from build123d import *

# Parameters (mm, degrees)
BOSS_EXTRUDE1_DEPTH              = 7.62
SKETCH2_W                        = 15.24
SKETCH2_H                        = 10.31875
CUT_EXTRUDE1_DEPTH               = 2.38125
SKETCH4_W                        = 10.31875
SKETCH4_H                        = 15.24
CUT_EXTRUDE2_DEPTH               = 2.38125
CHAMFER1_SIZE                    = 5.08
F_11_32_0_34375_DIAMETER_HOLE1_D = 8.73125


with BuildPart() as part:
    # Sketch1 → Boss-Extrude1 (new body, symmetric)
    with BuildSketch(Plane.XY):
        Polygon((0, 0), (0, 25.4), (6.35, 25.4), (6.35, 6.35), (25.4, 6.35), (25.4, 0), align=None)
    extrude(amount=BOSS_EXTRUDE1_DEPTH, both=True)

    # Sketch2 → Cut-Extrude1 (cut)
    with BuildSketch(Plane(origin=(6.35, 0, 0), x_dir=(0, 0, -1), z_dir=(1, 0, 0))):
        with Locations((0, 20.240625)):
            Rectangle(SKETCH2_W, SKETCH2_H)
    extrude(amount=-CUT_EXTRUDE1_DEPTH, mode=Mode.SUBTRACT)

    # Sketch4 → Cut-Extrude2 (cut)
    with BuildSketch(Plane(origin=(0, 6.35, 0), x_dir=(1, 0, 0), z_dir=(0, 1, 0))):
        with Locations((20.240625, 0)):
            Rectangle(SKETCH4_W, SKETCH4_H)
    extrude(amount=-CUT_EXTRUDE2_DEPTH, mode=Mode.SUBTRACT)

    # Chamfer1
    chamfer1_edges = [part.edges().sort_by_distance(p)[0] for p in [
        (0, 0, 0),
    ]]
    chamfer(chamfer1_edges, length=CHAMFER1_SIZE)

    # 11/32 (0.34375) Diameter Hole1 (through all)
    with Locations(Plane(origin=(2.54, 2.54, 0), x_dir=(0, 0, 1), z_dir=(-0.707106781, -0.707106781, 0))):
        with Locations((0, 0)):
            Hole(F_11_32_0_34375_DIAMETER_HOLE1_D / 2)


solid = part.part
For this review, take the finished solid that the model builds, in its own axes (mm). A direction names the side the tool comes from. Round coordinates to 2 decimals unless told otherwise and drop trailing zeros. Order: outer loops, then holes, each group sorted by start corner. A loop starts at its lowest first (then second) coordinate and runs counter-clockwise, first axis right, second up. Notation, with made-up numbers: (-4, 25) -> (46, 25) arc R16 cw to (46, 38) -> close; hole circle Ø7 at (15.5, 36.5). An arc over 180 degrees is marked (long way). Write item = value, one per line. Start each with the question number.
1) The part is to be moulded in two halves that separate along Y. For faces 3 (the face through (2.58, 2.5, -5.66)), 4 (the face through (2.224, 8.346, 0.568)), 5 (the face through (15.081, 5, 0)), say which applies: +Y half, -Y half, draft (parallel to the pull), parting line (faces both ways), or undercut.
2) Take a section at A-A on z = 5.25. State the section outline as (x, y) points.
3) Tool access review of faces 1 (the face through (20, 3.969, 0)), 2 (the face through (2.58, 2.5, 5.59)): name each direction out of +Z, -Z, +X, -X, +Y, -Y from which nothing blocks a thin tool from reaching the whole face with its end or side.
4) Take a section at C-C on y = 21. State the section outline as (x, z) points, plus the area to 3 significant figures.
5) To check wall thickness, follow line 1 (Y direction, x = 17, z = -3.25); line 2 (X direction, y = 13.5, z = 2.75). State the ranges of each line that lie inside material, in increasing order. Write a range as from..to.
6) Take a section at B-B on z = -0.25. State the section outline as (x, y) points, plus the area to 3 significant figures.
7) Insertion check: pin 1 (2 mm diameter, centred on x = 13.5, y = 7, fed in from +Z); pin 2 (1 mm diameter, centred on y = 5, z = 0.5, fed in from -X); pin 3 (2.5 mm diameter, centred on x = 9.5, z = -1, fed in from +Y); pin 4 (1.5 mm diameter, centred on x = 14.5, z = -5, fed in from +Y). Each pin has a flat end and moves straight along its axis. Give the tip position at first contact, or say it passes through.
Verdict:
q1.face_3 = -Y half
q1.face_4 = undercut
q1.face_5 = draft
q2.outline = (0, 5.08) -> (5.08, 0) -> (25.4, 0) -> (25.4, 3.97) -> (15.08, 3.97) -> (15.08, 6.35) -> (6.35, 6.35) -> (6.35, 15.08) -> (3.97, 15.08) -> (3.97, 25.4) -> (0, 25.4) -> close
q3.face_1 = +Z, -Z, +X, +Y
q3.face_2 = +Z, -Z, -X, -Y
q4.outline = (0, -7.62) -> (3.97, -7.62) -> (3.97, 7.62) -> (0, 7.62) -> close
q4.area = 60.5 mm2
q5.line_1 = 0..3.97
q5.line_2 = 0..6.35
q6.outline = (0, 6.16) -> (6.35, 12.51) -> (6.35, 15.08) -> (3.97, 15.08) -> (3.97, 25.4) -> (0, 25.4) -> close; (6.16, 0) -> (25.4, 0) -> (25.4, 3.97) -> (15.08, 3.97) -> (15.08, 6.35) -> (12.51, 6.35) -> close
q6.area = 155 mm2
q7.pin_1 = 7.62
q7.pin_2 = 10.63
q7.pin_3 = 4.85
q7.pin_4 = 6.35
